For this review, use the dimensioned drawing (mm, ordinates from the lowest corner) and the shaded views. A direction names the side the tool comes from. Coordinates: 2 decimals unless noted, no trailing zeros. Order: outer loops, then holes, each group sorted by start corner. A loop starts at its lowest first (then second) coordinate and runs counter-clockwise, first axis right, second up. Notation, with made-up numbers: M -3,-32.75 L 53,-32.75 A23 cw 53,-6.75 Z; hole C 57.5,41.5 d1. An arc over 180 degrees is marked long. Answer in a Markdown table with one row per item.
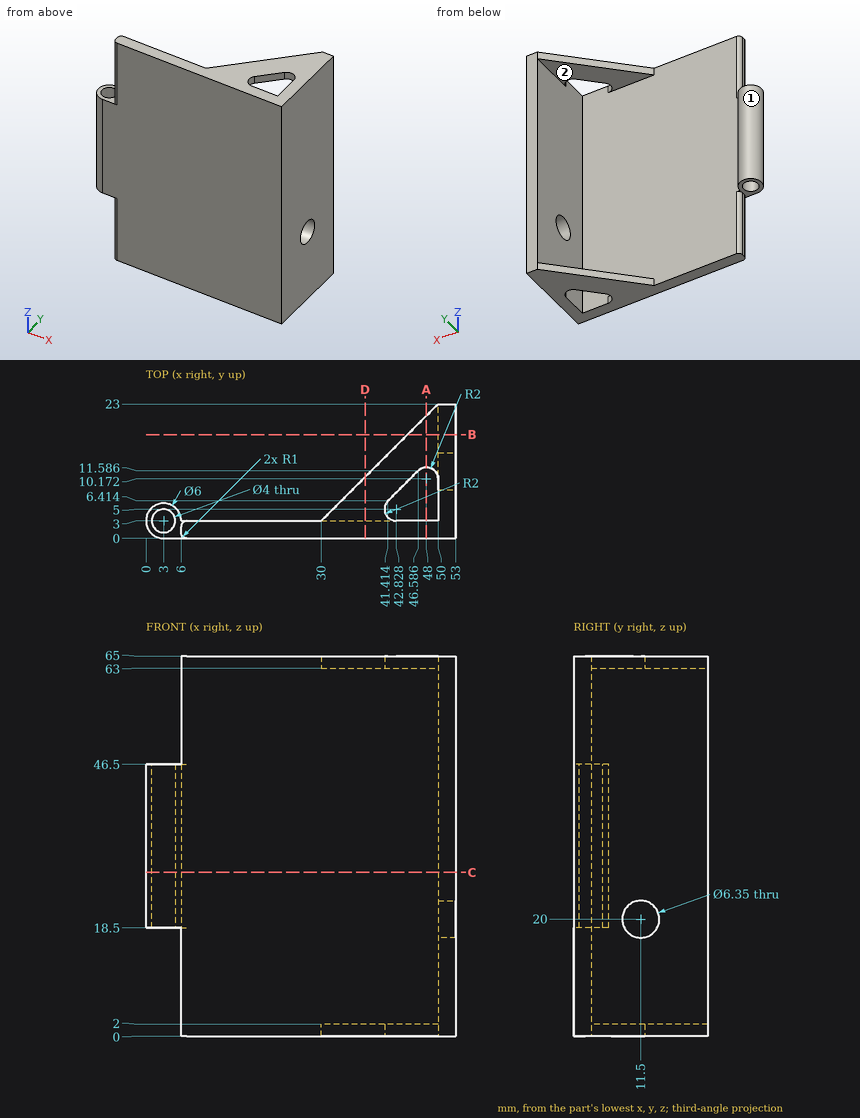
(1) Insertion check: P1, Ø12, axis at y = 14.5, z = 58, coming from the -X side (1 decimal); P2, Ø1, axis at y = 10, z = 45.5, coming from the -X side; P3, Ø10, axis at x = 35, z = 45, coming from the +Y side; P4, Ø4, axis at y = 11.5, z = 20, coming from the -X side. Each pin has a flat end and moves straight along its axis. Give the tip position at first contact, or say it passes through.
Report:
| item | result |
|---|---|
| P1 | x = 38.2 |
| P2 | x = 50 |
| P3 | y = 3 |
| P4 | through |
(2) Take a section at B-B (y = 17.75). Write out the cut boundary in (x, z).
Report:
| item | result |
|---|---|
| outline | M 44.75,0 L 53,0 L 53,65 L 44.75,65 L 44.75,63 L 50,63 L 50,2 L 44.75,2 Z |
(3) To check wall thickness, follow line 1 (Y direction, x = 3, z = 31); line 2 (Y direction, x = 51.3, z = 20) (1 decimal); line 3 (Z direction, x = 46, y = 14.25). State the ranges of each line that lie inside material, in increasing order. Write a range as [from, to].
Report:
| item | result |
|---|---|
| line 1 | [0, 1], [5, 6] |
| line 2 | [0, 8.3], [14.7, 23] |
| line 3 | [0, 2], [63, 65] |
(4) Machinability: for the marked faces 1 and 2, which of the approach directions +Z, -Z, +X, -X, +Y, -Y give a long, thin tool a straight path to every point of the face, cutting with its end or side? Answer none if there is none.
Report:
| item | result |
|---|---|
| face 1 | +Z, -Z |
| face 2 | -X, +Y |
(5) Take a section at A-A (x = 48). Write out the cut boundary in (y, z), then the cut area to 3 significant figures.
Report:
| item | result |
|---|---|
| outline | M 0,0 L 3,0 L 3,65 L 0,65 Z; M 12.17,0 L 21,0 L 21,2 L 12.17,2 Z; M 12.17,63 L 21,63 L 21,65 L 12.17,65 Z |
| area | 230 mm^2 |
(6) Take a section at C-C (z = 28). Write out the cut boundary in (x, y).
Report:
| item | result |
|---|---|
| outline | M 3,0 L 53,0 L 53,23 L 50,23 L 50,3 L 6,3 A3 ccw long Z; hole C 3,3 d4 |
(7) Take a section at D-D (x = 37.5). Write out the cut boundary in (y, z), then the cut area to 3 significant figures.
Report:
| item | result |
|---|---|
| outline | M 0,0 L 10.5,0 L 10.5,2 L 3,2 L 3,63 L 10.5,63 L 10.5,65 L 0,65 Z |
| area | 225 mm^2 |
